```python
from build123d import *

# Parameters (mm, degrees)
SKETCH1_R           = 31.5
SKETCH1_R_2         = 16
BOSS_EXTRUDE1_DEPTH = 14
SKETCH1_3_R         = 16
SKETCH1_3_R_2       = 12.5
SKETCH1_3_R_3       = 9
BOSS_EXTRUDE2_DEPTH = 8
SKETCH1_4_R         = 12.5
SKETCH1_4_R_2       = 9
BOSS_EXTRUDE3_DEPTH = 1
SKETCH2_R           = 3
CUT_EXTRUDE1_DEPTH  = 16
CUT_EXTRUDE2_DEPTH  = 6
SKETCH2_4_R         = 5
CUT_EXTRUDE3_DEPTH  = 11


with BuildPart() as part:
    # Sketch1 → Boss-Extrude1 (new body)
    with BuildSketch(Plane.XY):
        Circle(SKETCH1_R)
        Circle(SKETCH1_R_2, mode=Mode.SUBTRACT)
    extrude(amount=BOSS_EXTRUDE1_DEPTH)

    # Sketch1<3> → Boss-Extrude2 (add)
    with BuildSketch(Plane.XY):
        Circle(SKETCH1_3_R)
        Circle(SKETCH1_3_R_2, mode=Mode.SUBTRACT)
        Circle(SKETCH1_3_R_2)
        Circle(SKETCH1_3_R_3, mode=Mode.SUBTRACT)
    extrude(amount=BOSS_EXTRUDE2_DEPTH)

    # Sketch1<4> → Boss-Extrude3 (add)
    with BuildSketch(Plane.XY):
        Circle(SKETCH1_4_R)
        Circle(SKETCH1_4_R_2, mode=Mode.SUBTRACT)
    extrude(amount=-BOSS_EXTRUDE3_DEPTH)

    # Sketch2 → Cut-Extrude1 (cut, through all)
    with BuildSketch(Plane.XY.offset(14)):
        with Locations((-20, 0)):
            Circle(SKETCH2_R)
        with Locations((0, 20)):
            Circle(SKETCH2_R)
        with Locations((20, 0)):
            Circle(SKETCH2_R)
        with Locations((0, -20)):
            Circle(SKETCH2_R)
    extrude(amount=-CUT_EXTRUDE1_DEPTH, mode=Mode.SUBTRACT)

    # Sketch2<3> → Cut-Extrude2 (cut)
    with BuildSketch(Plane.XY.offset(14)):
        with BuildLine():
            Line((-20, -5), (-15.198684154, -5))
            ThreePointArc((-15.198684154, -5), (-15.53045532, -3.847721084), (-15.775, -2.67383152))
            ThreePointArc((-15.775, -2.67383152), (-17.588481557, -4.380020411), (-20, -5))
        make_face()
        with BuildLine():
            ThreePointArc((-20, 5), (-17.588481557, 4.380020411), (-15.775, 2.67383152))
            ThreePointArc((-15.775, 2.67383152), (-15.53045532, 3.847721084), (-15.198684154, 5))
            Line((-15.198684154, 5), (-20, 5))
        make_face()
        with BuildLine():
            Line((-5, 20), (-5, 15.198684154))
            ThreePointArc((-5, 15.198684154), (-3.847721084, 15.53045532), (-2.67383152, 15.775))
            ThreePointArc((-2.67383152, 15.775), (-4.380020411, 17.588481557), (-5, 20))
        make_face()
        with BuildLine():
            Line((5, 15.198684154), (5, 20))
            ThreePointArc((5, 20), (4.380020411, 17.588481557), (2.67383152, 15.775))
            ThreePointArc((2.67383152, 15.775), (3.847721084, 15.53045532), (5, 15.198684154))
        make_face()
        with BuildLine():
            ThreePointArc((-2.67383152, -15.775), (-3.847721084, -15.53045532), (-5, -15.198684154))
            Line((-5, -15.198684154), (-5, -20))
            ThreePointArc((-5, -20), (-4.380020411, -17.588481557), (-2.67383152, -15.775))
        make_face()
        with BuildLine():
            ThreePointArc((2.67383152, -15.775), (4.380020411, -17.588481557), (5, -20))
            Line((5, -20), (5, -15.198684154))
            ThreePointArc((5, -15.198684154), (3.847721084, -15.53045532), (2.67383152, -15.775))
        make_face()
        with BuildLine():
            ThreePointArc((15.775, -2.67383152), (15.53045532, -3.847721084), (15.198684154, -5))
            Line((15.198684154, -5), (20, -5))
            ThreePointArc((20, -5), (17.588481557, -4.380020411), (15.775, -2.67383152))
        make_face()
        with BuildLine():
            Line((20, 5), (15.198684154, 5))
            ThreePointArc((15.198684154, 5), (15.53045532, 3.847721084), (15.775, 2.67383152))
            ThreePointArc((15.775, 2.67383152), (17.588481557, 4.380020411), (20, 5))
        make_face()
    extrude(amount=-CUT_EXTRUDE2_DEPTH, mode=Mode.SUBTRACT)

    # Sketch2<4> → Cut-Extrude3 (cut)
    with BuildSketch(Plane.XY.offset(14)):
        with Locations((-20, 0)):
            Circle(SKETCH2_4_R)
        with Locations((20, 0)):
            Circle(SKETCH2_4_R)
        with Locations((0, 20)):
            Circle(SKETCH2_4_R)
        with Locations((0, -20)):
            Circle(SKETCH2_4_R)
    extrude(amount=-CUT_EXTRUDE3_DEPTH, mode=Mode.SUBTRACT)


solid = part.part
```
For this review, take the finished solid that the model builds, in its own axes (mm). A direction names the side the tool comes from. Round coordinates to 2 decimals unless told otherwise and drop trailing zeros. Write each loop counter-clockwise with the first axis right and the second up, starting at its lowest first coordinate (ties: lowest second). Pieces come first, ordered by that corner, then holes. Notation, with made-up numbers: (42, -3.5) - (77, -3.5) arc R20 cw to (77, 13.5) - close; hole circle Ø7 at (-10.75, 58.5). An arc over 180 degrees is marked (long way). Answer as a JSON object with one key per item and string values.
1. We need section D-D on x = 19. Give the boundary of the cut face in (y, z).
Response values:
{"outline": "(-25.12, 0) - (-2.83, 0) - (-2.83, 3) - (-4.9, 3) - (-4.9, 8) - (-5, 8) - (-5, 14) - (-25.12, 14) - close; (2.83, 0) - (25.12, 0) - (25.12, 14) - (5, 14) - (5, 8) - (4.9, 8) - (4.9, 3) - (2.83, 3) - close"}
2. We need section A-A on z = 12.75. Give the boundary of the cut face in (x, y).
Response values:
{"outline": "circle Ø63 at (0, 0); hole (-20, -5) - (-15.2, -5) arc R16 ccw to (-5, -15.2) - (-5, -20) arc R5 ccw to (5, -20) - (5, -15.2) arc R16 ccw to (15.2, -5) - (20, -5) arc R5 ccw to (20, 5) - (15.2, 5) arc R16 ccw to (5, 15.2) - (5, 20) arc R5 ccw to (-5, 20) - (-5, 15.2) arc R16 ccw to (-15.2, 5) - (-20, 5) arc R5 ccw to start"}
3. Draft analysis for pull direction Y (two halves, no side actions). For faces 3 (the face through (-9, 3, -1)), 4 (the face through (18, -5, 11)), 5 (the face through (-4.101, 31.232, 6.902)), state which applies: +Y half, -Y half, draft (parallel to the pull), parting line (faces both ways), or undercut.
Response values:
{"face 3": "draft", "face 4": "undercut", "face 5": "parting line"}
4. We need section C-C on z = 2.25. Give the boundary of the cut face in (x, y), then the cut area to 3 significant figures.
Response values:
{"outline": "circle Ø63 at (0, 0); hole circle Ø6 at (-20, 0); hole circle Ø18 at (0, 0); hole circle Ø6 at (0, -20); hole circle Ø6 at (0, 20); hole circle Ø6 at (20, 0)", "area": "2,750 mm2"}
5. For pin 1 Ø2 at (y, z) = (0.5, 6.5) entering from +X; pin 2 Ø1.5 at (x, y) = (-21, 11) entering from -Z; pin 3 Ø1.4 at (y, z) = (-17.5, 11) entering from +X; pin 4 Ø12 at (x, y) = (6, 5) entering from +Z, all flat-tipped, find the tip position at first contact; note any pin that passes through.
Response values:
{"pin 1": "stops at x = 31.5", "pin 2": "stops at z = 0", "pin 3": "stops at x = 26.65", "pin 4": "stops at z = 8"}
6. Tool access review of faces 1 (the face through (-11.388, -11.239, 10.958)), 2 (the face through (17, 0, 2)): name each direction out of +Z, -Z, +X, -X, +Y, -Y from which nothing blocks a thin tool from reaching the whole face with its end or side.
Response values:
{"face 1": "+Z", "face 2": "+Z, -Z"}
7. To check wall thickness, follow line 1 along Y through (x, z) = (0, 4.25); line 2 along Y through (x, z) = (0, 2); line 3 along Y through (x, z) = (0, -0.75). State the ranges of each line that lie inside material, in increasing order.
Response values:
{"line 1": "y = -31.5 to -25, -15 to -9, 9 to 15, 25 to 31.5", "line 2": "y = -31.5 to -23, -17 to -9, 9 to 17, 23 to 31.5", "line 3": "y = -12.5 to -9, 9 to 12.5"}
8. We need section B-B on x = 0. Give the boundary of the cut face in (y, z), then the cut area to 3 significant figures.
Response values:
{"outline": "(-31.5, 0) - (-23, 0) - (-23, 3) - (-25, 3) - (-25, 14) - (-31.5, 14) - close; (-17, 0) - (-12.5, 0) - (-12.5, -1) - (-9, -1) - (-9, 8) - (-15, 8) - (-15, 3) - (-17, 3) - close; (9, -1) - (12.5, -1) - (12.5, 0) - (17, 0) - (17, 3) - (15, 3) - (15, 8) - (9, 8) - close; (23, 0) - (31.5, 0) - (31.5, 14) - (25, 14) - (25, 3) - (23, 3) - close", "area": "309 mm2"}
